Input: part model. Units: mm. Frame: model coordinates. A direction names the side the tool comes from. Coordinates: 2 decimals unless noted, no trailing zeros. Loops run counter-clockwise (first coordinate to the right, second up) from the corner with the lowest first, then second, coordinate; pieces in that order, holes last.
```python
from build123d import *

# Parameters (mm, degrees)
SKETCH1_R             = 25
BOSS_EXTRUDE1_DEPTH   = 20
SKETCH2_W             = 38.5
SKETCH2_H             = 19.05
BOSS_EXTRUDE2_DEPTH   = 5.4
M10_CLEARANCE_HOLE1_D = 11


with BuildPart() as part:
    # Sketch1 → Boss-Extrude1 (new body)
    with BuildSketch(Plane.XY):
        with BuildLine():
            Line((-76.2, -25), (-76.2, -44.05))
            Line((-76.2, -44.05), (76.2, -44.05))
            Line((76.2, -44.05), (76.2, -25))
            Line((76.2, -25), (37.7, -25))
            Line((37.7, -25), (37.7, 0))
            ThreePointArc((37.7, 0), (0, 37.7), (-37.7, 0))
            Line((-37.7, 0), (-37.7, -25))
            Line((-37.7, -25), (-76.2, -25))
        make_face()
        Circle(SKETCH1_R, mode=Mode.SUBTRACT)
    extrude(amount=BOSS_EXTRUDE1_DEPTH)

    # Sketch2 → Boss-Extrude2 (add)
    with BuildSketch(Plane.XY.offset(20)):
        with Locations((-56.95, -34.525)):
            Rectangle(SKETCH2_W, SKETCH2_H)
        with Locations((56.95, -34.525)):
            Rectangle(SKETCH2_W, SKETCH2_H)
    extrude(amount=BOSS_EXTRUDE2_DEPTH)

    # M10 Clearance Hole1 (through all)
    with Locations(Plane(origin=(0, -25, 0), x_dir=(1, 0, 0), z_dir=(0, 1, 0))):
        with Locations((-57.2, -12.7), (57.2, -12.7)):
            Hole(M10_CLEARANCE_HOLE1_D / 2)


solid = part.part
```
Item 1: Reachability of faces 5 (the face through (62.695, -34.658, 12.458)), 6 (the face through (-76.2, -35, 13)), 7 (the face through (37.7, -35, 23)), 8 (the face through (-37.7, -12, 10)), 9 (the face through (37.7, -13, 10)) from +Z, -Z, +X, -X, +Y, -Y: full face, straight path, thin tool, end or side. Return the list, or none.
Result:
face 5: +Y, -Y
face 6: +Z, -Z, -X, +Y, -Y
face 7: +Z, +Y, -Y
face 8: +Z, -Z, -X, +Y
face 9: +Z, -Z, +X, +Y
Item 2: Mould query, pull axis Y, two halves, no side actions, for faces 1 (the face through (57, -34, 25.4)), 2 (the face through (23.846, 7.509, 9.86)), 3 (the face through (-1, -44.05, 13)), 4 (the face through (0.83, 37.69, 9.86)). Classes: +Y half, -Y half, draft (parallel to the pull), parting line (faces both ways), or undercut.
Result:
face 1: draft
face 2: undercut
face 3: -Y half
face 4: +Y half
Item 3: Section query C-C (z = 9). Output: boundary loops of the cut face in (x, y), then the cut area to 3 significant figures.
Result:
outline: (-76.2, -44.05) - (-61.27, -44.05) - (-61.27, -25) - (-76.2, -25) - close; (-53.13, -44.05) - (53.13, -44.05) - (53.13, -25) - (37.7, -25) - (37.7, 0) arc R37.7 ccw to (-37.7, 0) - (-37.7, -25) - (-53.13, -25) - close; (61.27, -44.05) - (76.2, -44.05) - (76.2, -25) - (61.27, -25) - close; hole circle Ø50 at (0, 0)
area: 4,750 mm2
Item 4: Section query A-A (y = -20). Output: boundary loops of the cut face in (x, z).
Result:
outline: (-37.7, 0) - (-15, 0) - (-15, 20) - (-37.7, 20) - close; (15, 0) - (37.7, 0) - (37.7, 20) - (15, 20) - close
Item 5: Line query: L1, parallel to Z at x = 57.2, y = -38.75; L2, parallel to Y at x = 42.5, z = 20.25; L3, parallel to Y at x = 0, z = 13. Output: solid intervals per line, ascending.
Result:
L1: z = 0 to 7.2, 18.2 to 25.4
L2: y = -44.05 to -25
L3: y = -44.05 to -25, 25 to 37.7
Item 6: Section query D-D (y = -28.5). Output: boundary loops of the cut face in (x, z).
Result:
outline: (-76.2, 0) - (76.2, 0) - (76.2, 25.4) - (37.7, 25.4) - (37.7, 20) - (-37.7, 20) - (-37.7, 25.4) - (-76.2, 25.4) - close; hole circle Ø11 at (-57.2, 12.7); hole circle Ø11 at (57.2, 12.7)
Item 7: Section query B-B (x = 0). Output: boundary loops of the cut face in (y, z).
Result:
outline: (-44.05, 0) - (-25, 0) - (-25, 20) - (-44.05, 20) - close; (25, 0) - (37.7, 0) - (37.7, 20) - (25, 20) - close
Item 8: Contact query for flat-ended pins moving along their axis: P1, Ø12.5, axis at x = 59, z = 17.5, coming from the +Y side; P2, Ø6, axis at y = -13.5, z = 10, coming from the +X side; P3, Ø2, axis at x = -26.5, y = 22, coming from the +Z side. Output: stop coordinate, or through.
Result:
P1: stops at y = -25
P2: stops at x = 37.7
P3: stops at z = 20
